from build123d import *

# Parameters (mm, degrees)
FILLET1_R    = 0.1
RECPAT_COUNT = 2
RECPAT_ANGLE = 90
SCHIZZO1_W   = 0.5
SCHIZZO1_H   = 4


with BuildPart() as part:
    # BodySke → Base-Revolve (revolve)
    with BuildSketch(Plane.XY, mode=Mode.PRIVATE) as base_revolve_sk:
        with BuildLine():
            Line((2.4, 1.5), (2.4, 2.8))
            Line((2.4, 2.8), (1.003501533, 2.8))
            ThreePointArc((1.003501533, 2.8), (0.873295971, 2.76653015), (0.775371599, 2.674418605))
            ThreePointArc((0.775371599, 2.674418605), (0.197753546, 1.392274756), (0, 0))
            Line((0, 0), (10.4, 0))
            Line((10.4, 0), (10.4, 1.5))
            Line((10.4, 1.5), (2.4, 1.5))
        make_face()
    revolve(base_revolve_sk.sketch.rotate(Axis((1.003501533, 0, 0), (1, 0, 0)), 90), axis=Axis((1.003501533, 0, 0), (1, 0, 0)))

    # Fillet1
    fillet1_edges = [part.edges().sort_by_distance(p)[0] for p in [
        (2.4, 0, -1.5),
    ]]
    fillet(fillet1_edges, radius=FILLET1_R)

    # Sketch3 → Recess section 0
    with BuildSketch(Plane(origin=(0, 0, 0), x_dir=(0, 0, -1), z_dir=(1, 0, 0))):
        with BuildLine():
            Line((0.37, -1.4), (-0.37, -1.4))
            Line((-0.37, -1.4), (-0.37, 1.4))
            Line((-0.37, 1.4), (0.37, 1.4))
            Line((0.37, 1.4), (0.37, -1.4))
        make_face()
    # Sketch4 → Recess section 1
    with BuildSketch(Plane(origin=(1.75, 0, 0), x_dir=(0, 0, -1), z_dir=(1, 0, 0))):
        with BuildLine():
            Line((0.37, -0.527482332), (-0.37, -0.527482332))
            Line((-0.37, -0.527482332), (-0.37, 0.527482332))
            Line((-0.37, 0.527482332), (0.37, 0.527482332))
            Line((0.37, 0.527482332), (0.37, -0.527482332))
        make_face()
    recess = loft(mode=Mode.SUBTRACT)

    # RecPat: Recess ×2 about axis
    recpat_axis = Axis((0, 0, 0), (1, 0, 0))
    for i in range(1, RECPAT_COUNT):
        add(recess.rotate(recpat_axis, i * RECPAT_ANGLE / (RECPAT_COUNT - 1)), mode=Mode.SUBTRACT)

    # RecCorSke → RecessCore (revolve, cut)
    with BuildSketch(Plane.XY, mode=Mode.PRIVATE) as recesscore_sk:
        Polygon((0, 0), (0, 0.678371921), (1.75, 0.556), (1.930655351, 0), align=None)
    revolve(recesscore_sk.sketch.rotate(Axis((-3.175, 0, 0), (1, 0, 0)), 15.814025638), axis=Axis((-3.175, 0, 0), (1, 0, 0)), mode=Mode.SUBTRACT)

    # Schizzo1 → Rivoluzione2 (revolve)
    with BuildSketch(Plane(origin=(0, 0, 0), x_dir=(1, 0, 0), z_dir=(0, 1, 0))):
        with Locations((2.15, -2)):
            Rectangle(SCHIZZO1_W, SCHIZZO1_H)
    revolve(axis=Axis((0, 0, 0), (1, 0, 0)))


solid = part.part
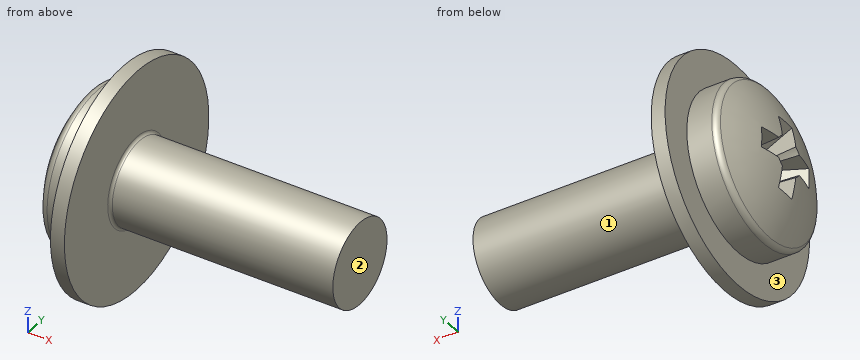
Read the model definition and answer for the solid it produces. Units are mm, in the model's axes. Face numbers are marked on the shaded views. A direction names the side the tool comes from. Coordinates: 2 decimals unless noted, no trailing zeros. Write each loop counter-clockwise with the first axis right and the second up, starting at its lowest first coordinate (ties: lowest second). Pieces come first, ordered by that corner, then holes. Notation, with made-up numbers: M 57,89 L 70,89 A25 cw 70,127 Z; hole C -38,7 d10. An arc over 180 degrees is marked long. Use a Markdown table: item, result.
Q1. Each of these flat-tipped pins is pushed along its axis until it touches: pin 1 Ø2 at (x, z) = (8.5, -1) entering from +Y; pin 2 Ø3 at (x, y) = (1.5, -2.5) entering from +Z; pin 3 Ø2 at (x, y) = (8.5, -0.5) entering from -Z; pin 4 Ø2.5 at (y, z) = (-0.5, -1.5) entering from -X. Where does it stop, or does it pass through?
Answer block:
| item | result |
|---|---|
| pin 1 | stops at y = 1.5 |
| pin 2 | stops at z = 3.86 |
| pin 3 | stops at z = -1.5 |
| pin 4 | stops at x = 0.05 |
Q2. Which of the six approach directions +Z, -Z, +X, -X, +Y, -Y give full straight-line access (tool end or side, diameter ignored) to the marked faces 1, 2 and 3?
Answer block:
| item | result |
|---|---|
| face 1 | +X |
| face 2 | +Z, -Z, +X, +Y, -Y |
| face 3 | -X |
Q3. Straight lines are drawn through the part: L1, parallel to X at y = -0.75, z = 3.75; L2, parallel to X at y = 0.5, z = 0.5; L3, parallel to Y at x = 8.5, z = -1.25. For each, find the intervals that lie inside material, in ascending order. Write a range as [from, to].
Answer block:
| item | result |
|---|---|
| L1 | x = [1.9, 2.4] |
| L2 | x = [0.05, 10.4] |
| L3 | y = [-0.83, 0.83] |
Q4. The part is cut by section A-A, the plane x = 5. Write down the section's boundary in (y, z).
Answer block:
| item | result |
|---|---|
| outline | C 0,0 d3 |
